Can you work these out from the model? Positions are in its coordinate system, mm. Face numbers are marked on the shaded views. A direction names the side the tool comes from. Coordinates: 2 decimals unless noted, no trailing zeros. Order: outer loops, then holes, each group sorted by start corner. A loop starts at its lowest first (then second) coordinate and runs counter-clockwise, first axis right, second up.
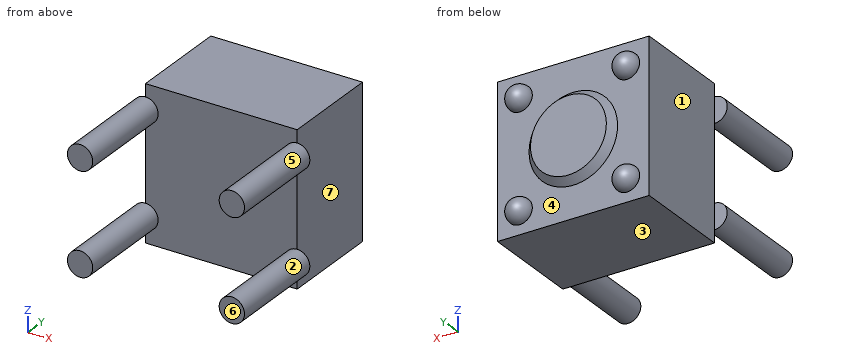
```python
from build123d import *

# Parameters (mm, degrees)
SKETCH1_W           = 6
SKETCH1_H           = 6
BOSS_EXTRUDE1_DEPTH = 4
BOSS_EXTRUDE2_START = -4
SKETCH2_R           = 1.75
BOSS_EXTRUDE2_DEPTH = 4.3
SKETCH4_R           = 0.5
BOSS_EXTRUDE3_DEPTH = 0.5
FILLET1_R           = 0.5
SKETCH5_R           = 0.5
BOSS_EXTRUDE4_DEPTH = 4


with BuildPart() as part:
    # Sketch1 → Boss-Extrude1 (new body)
    with BuildSketch(Plane(origin=(0, 0, 0), x_dir=(1, 0, 0), z_dir=(0, 1, 0))):
        Rectangle(SKETCH1_W, SKETCH1_H)
    extrude(amount=BOSS_EXTRUDE1_DEPTH)

    # Sketch2 → Boss-Extrude2 (add)
    with BuildSketch(Plane(origin=(0, 4, 0), x_dir=(1, 0, 0), z_dir=(0, 1, 0)).offset(BOSS_EXTRUDE2_START)):
        with Locations(Location((0, 0, 0), (0, 0, 90))):
            Circle(SKETCH2_R)
    extrude(amount=BOSS_EXTRUDE2_DEPTH)

    # Sketch3 → Cut-Revolve1 (revolve, cut)
    with BuildSketch(Plane(origin=(0, 0, 0), x_dir=(0, 0, -1), z_dir=(1, 0, 0))):
        Polygon((-1.75, 4.3), (-1.75, 4), (-1.5, 4.3), align=None)
    revolve(axis=Axis((0, 8.374446569, 0), (0, -1, 0)), mode=Mode.SUBTRACT)

    # Sketch4 → Boss-Extrude3 (add)
    with BuildSketch(Plane(origin=(0, 4, 0), x_dir=(1, 0, 0), z_dir=(0, 1, 0))):
        with Locations(Location((-2.121320344, 2.121320344, 0), (0, 0, 270))):
            Circle(SKETCH4_R)
        with Locations(Location((2.121320344, 2.121320344, 0), (0, 0, 270))):
            Circle(SKETCH4_R)
        with Locations(Location((2.121320344, -2.121320344, 0), (0, 0, 270))):
            Circle(SKETCH4_R)
        with Locations(Location((-2.121320344, -2.121320344, 0), (0, 0, 270))):
            Circle(SKETCH4_R)
    extrude(amount=BOSS_EXTRUDE3_DEPTH)

    # Fillet1
    fillet1_edges = [part.edges().sort_by_distance(p)[0] for p in [
        (-2.121320344, 4.5, -2.621320344),
        (2.121320344, 4.5, -2.621320344),
        (2.121320344, 4.5, 1.621320344),
        (-2.121320344, 4.5, 1.621320344),
    ]]
    fillet(fillet1_edges, radius=FILLET1_R - 0.0001)  # a hair under: the kernel refuses the full size

    # Sketch5 → Boss-Extrude4 (add)
    with BuildSketch(Plane(origin=(0, 0, 0), x_dir=(1, 0, 0), z_dir=(0, 1, 0))):
        with Locations(Location((3, -2, 0), (0, 0, 270))):
            Circle(SKETCH5_R)
        with Locations(Location((3, 2, 0), (0, 0, 90))):
            Circle(SKETCH5_R)
        with Locations(Location((-3, 2, 0), (0, 0, 270))):
            Circle(SKETCH5_R)
        with Locations(Location((-3, -2, 0), (0, 0, 90))):
            Circle(SKETCH5_R)
    extrude(amount=-BOSS_EXTRUDE4_DEPTH)


solid = part.part
```
1. I'm going to push flat-ended pins straight in: pin 1 (2 mm diameter, centred on y = 2.5, z = 0, fed in from +X); pin 2 (0.9 mm diameter, centred on x = 0.5, z = 0, fed in from +Y); pin 3 (0.6 mm diameter, centred on x = 3, z = -2, fed in from +Y). Where does each tip first touch, or does it pass through?
Completed:
pin 1: stops at x = 3
pin 2: stops at y = 4.3
pin 3: stops at y = 4
2. Please list where these lines run through material, in increasing order: probe 1 along Y at (x, z) = (1.25, 1.9); probe 2 along X at (y, z) = (-2.75, 2.3); probe 3 along Y at (x, z) = (2, 2.5).
Completed:
probe 1: y = 0 to 4
probe 2: x = -3.4 to -2.6, 2.6 to 3.4
probe 3: y = 0 to 4.3
3. Thinking about a two-plate mould opening in X: for the marked faces 1, 2 and 3, which applies, pulls with the +X half, pulls with the -X half, needs draft (parallel to the pull), parting line crosses it, or undercut?
Completed:
face 1: pulls with the -X half
face 2: undercut
face 3: needs draft
4. Imagine slicing it at B-B on y = -3.5. Please give me the cut outline in (x, z), then the cut area to 3 significant figures.
Completed:
outline: circle Ø1 at (-3, -2); circle Ø1 at (-3, 2); circle Ø1 at (3, -2); circle Ø1 at (3, 2)
area: 3.14 mm2
5. Imagine slicing it at D-D on x = 2.75. Please give me the cut outline in (y, z), then the cut area to 3 significant figures.
Completed:
outline: (-4, -2.43) - (0, -2.43) - (0, -3) - (4, -3) - (4, 3) - (0, 3) - (0, 2.43) - (-4, 2.43) - (-4, 1.57) - (0, 1.57) - (0, -1.57) - (-4, -1.57) - close
area: 30.9 mm2
6. On a 3-axis mill with a long thin cutter (end or side, diameter ignored), from which of +Z, -Z, +X, -X, +Y, -Y can I reach the whole of each face in a straight line? I mean the marked faces 4, 5, 6 and 7. Say none if no direction works.
Completed:
face 4: +Y
face 5: -Y
face 6: +Z, -Z, +X, -X, -Y
face 7: +Z, -Z, +X, +Y
7. Imagine slicing it at C-C on y = 1. Please give me the cut outline in (x, z), then the cut area to 3 significant figures.
Completed:
outline: (-3, -3) - (3, -3) - (3, 3) - (-3, 3) - close
area: 36.0 mm2
8. Imagine slicing it at A-A on x = 0. Please give me the cut outline in (y, z), then the cut area to 3 significant figures.
Completed:
outline: (0, -3) - (4, -3) - (4, -1.75) - (4.3, -1.5) - (4.3, 1.5) - (4, 1.75) - (4, 3) - (0, 3) - close
area: 25.0 mm2
